from build123d import *

# Parameters (mm, degrees)
BASE_FLANGE1_DEPTH                 = 85.725
SKETCH2_R                          = 6.5532
SKETCH2_R_2                        = 3.3147
SKETCH2_R_3                        = 2.667
SKETCH2_R_4                        = 1.8669
FCE_1_INDICATOR_HOLES_DEPTH        = 2.54
SKETCH3_R                          = 2.1082
FCE_2_BRACKET_MOUNTING_HOLES_DEPTH = 2.54
CHAMFER1_SIZE                      = 1.27
SKETCH8_R                          = 2.1082
FCE_3_BOARD_MOUNTING_HOLES_DEPTH   = 2.54
FILLET1_R                          = 3.175


# Sheet-metal steps are written as plain solids
with BuildPart() as part:
    # Sketch1 → Base-Flange1 (new, symmetric)
    with BuildSketch(Plane(origin=(0, 0, 0), x_dir=(1, 0, 0), z_dir=(0, 1, 0))):
        with BuildLine():
            Line((-31.75, -101.6), (-3.302, -101.6))
            ThreePointArc((-3.302, -101.6), (-0.967133409, -100.632866591), (0, -98.298))
            Line((0, -98.298), (0, -3.302))
            ThreePointArc((0, -3.302), (-0.967133409, -0.967133409), (-3.302, 0))
            Line((-3.302, 0), (-53.975, 0))
            Line((-53.975, 0), (-53.975, -2.032))
            Line((-53.975, -2.032), (-3.302, -2.032))
            ThreePointArc((-3.302, -2.032), (-2.403974388, -2.403974388), (-2.032, -3.302))
            Line((-2.032, -3.302), (-2.032, -98.298))
            ThreePointArc((-2.032, -98.298), (-2.403974388, -99.196025612), (-3.302, -99.568))
            Line((-3.302, -99.568), (-31.75, -99.568))
            Line((-31.75, -99.568), (-31.75, -101.6))
        make_face()
    extrude(amount=BASE_FLANGE1_DEPTH, both=True)

    # Sketch2 → FCE-1 Indicator holes (cut)
    with BuildSketch(Plane(origin=(0, 0, 101.6), x_dir=(-1, 0, 0), z_dir=(0, 0, -1))):
        with Locations(Location((14.732, 63.5, 0), (0, 0, 180))):
            Circle(SKETCH2_R)
        with Locations(Location((14.732, 44.45, 0), (0, 0, 180))):
            Circle(SKETCH2_R)
        with Locations(Location((14.732, -12.7, 0), (0, 0, 180))):
            Circle(SKETCH2_R_2)
        with Locations(Location((18.034, -25.4, 0), (0, 0, 180))):
            Circle(SKETCH2_R_3)
        with Locations(Location((18.034, -38.1, 0), (0, 0, 180))):
            Circle(SKETCH2_R_3)
        with Locations(Location((18.034, -50.8, 0), (0, 0, 180))):
            Circle(SKETCH2_R_3)
        with Locations(Location((17.272, -63.5, 0), (0, 0, 180))):
            Circle(SKETCH2_R_4)
    extrude(amount=FCE_1_INDICATOR_HOLES_DEPTH, mode=Mode.SUBTRACT)

    # Sketch3 → FCE-2 Bracket Mounting Holes (cut)
    with BuildSketch(Plane.XY.offset(2.032)):
        with Locations((-44.45, 76.2)):
            Circle(SKETCH3_R)
        with Locations((-44.45, 0)):
            Circle(SKETCH3_R)
        with Locations((-44.45, -76.2)):
            Circle(SKETCH3_R)
    extrude(amount=-FCE_2_BRACKET_MOUNTING_HOLES_DEPTH, mode=Mode.SUBTRACT)

    # Chamfer1
    chamfer1_edges = [part.edges().sort_by_distance(p)[0] for p in [
        (-20.701, -25.4, 101.6),
        (-20.701, -38.1, 101.6),
        (-20.701, -50.8, 101.6),
    ]]
    chamfer(chamfer1_edges, length=CHAMFER1_SIZE)

    # Sketch8 → FCE-3 Board Mounting Holes (cut)
    with BuildSketch(Plane.ZY.offset(2.032)):
        with Locations((93.218, 76.2)):
            Circle(SKETCH8_R)
        with Locations((93.218, 0)):
            Circle(SKETCH8_R)
        with Locations((93.218, -76.2)):
            Circle(SKETCH8_R)
        with Locations((29.718, -76.2)):
            Circle(SKETCH8_R)
        with Locations((29.718, 0)):
            Circle(SKETCH8_R)
        with Locations((29.718, 76.2)):
            Circle(SKETCH8_R)
    extrude(amount=-FCE_3_BOARD_MOUNTING_HOLES_DEPTH, mode=Mode.SUBTRACT)

    # Fillet1
    fillet1_edges = [part.edges().sort_by_distance(p)[0] for p in [
        (-31.75, -85.725, 100.584),
        (-53.975, 85.725, 1.016),
        (-31.75, 85.725, 100.584),
        (-53.975, -85.725, 1.016),
    ]]
    fillet(fillet1_edges, radius=FILLET1_R)


solid = part.part
Can you work these out from the model? Positions are in its coordinate system, mm. A direction names the side the tool comes from. Coordinates: 2 decimals unless noted, no trailing zeros. Order: outer loops, then holes, each group sorted by start corner. A loop starts at its lowest first (then second) coordinate and runs counter-clockwise, first axis right, second up. Notation, with made-up numbers: M 18,-31.5 L 59,-31.5 A17 cw 59,-24.5 Z; hole C 73.25,23.25 d1. An arc over 180 degrees is marked long. Write item = value, one per line.
(1) Suppose I cut it at D-D on y = 44.45. Please give me the cut outline in (x, z) (3 decimals), plus the area to 3 significant figures.
Results are:
outline = M -53.975,0 L -3.302,0 A3.302 ccw 0,3.302 L 0,98.298 A3.302 ccw -3.302,101.6 L -8.179,101.6 L -8.179,99.568 L -3.302,99.568 A1.27 cw -2.032,98.298 L -2.032,3.302 A1.27 cw -3.302,2.032 L -53.975,2.032 Z; M -31.75,99.568 L -21.285,99.568 L -21.285,101.6 L -31.75,101.6 Z
area = 342 mm2
(2) For pin 1 Ø14 at (x, y) = (-14.5, -14) entering from -Z; pin 2 Ø3 at (x, y) = (-34, -65) entering from +Z; pin 3 Ø12 at (y, z) = (-39.5, 57.5) entering from -X; pin 4 Ø0.6 at (y, z) = (-22, 100.5) entering from -X, each with a flat end and sliding along its axis, tell me the tip position at first contact or that it passes through.
Results are:
pin_1 = 0
pin_2 = 2.03
pin_3 = -2.03
pin_4 = -31.75
(3) Suppose I cut it at A-A on y = 0. Please give me the cut outline in (x, z) (3 decimals).
Results are:
outline = M -53.975,0 L -46.558,0 L -46.558,2.032 L -53.975,2.032 Z; M -42.342,0 L -3.302,0 A3.302 ccw 0,3.302 L 0,27.61 L -2.032,27.61 L -2.032,3.302 A1.27 cw -3.302,2.032 L -42.342,2.032 Z; M -31.75,99.568 L -3.302,99.568 A1.27 cw -2.032,98.298 L -2.032,95.326 L 0,95.326 L 0,98.298 A3.302 ccw -3.302,101.6 L -31.75,101.6 Z; M -2.032,31.826 L 0,31.826 L 0,91.11 L -2.032,91.11 Z
(4) Suppose I cut it at C-C on x = -38.5. Please give me the cut outline in (y, z) (3 decimals), plus the area to 3 significant figures.
Results are:
outline = M -85.725,0 L 85.725,0 L 85.725,2.032 L -85.725,2.032 Z
area = 348 mm2
(5) If we mould it in two halves opening along X, with no side actions, what happens to faces 1 (the face through (-2.032, 1, 50)), 2 (the face through (-42.44, 0.63, 1.03)), 3 (the face through (-17, 1, 99.568))? For each: pulls with the +X half, pulls with the -X half, needs draft (parallel to the pull), parting line crosses it, or undercut.
Results are:
face_1 = pulls with the -X half
face_2 = undercut
face_3 = needs draft
(6) Suppose I cut it at B-B on y = -50.8. Please give me the cut outline in (x, z) (3 decimals).
Results are:
outline = M -53.975,0 L -3.302,0 A3.302 ccw 0,3.302 L 0,98.298 A3.302 ccw -3.302,101.6 L -14.097,101.6 L -15.367,100.33 L -15.367,99.568 L -3.302,99.568 A1.27 cw -2.032,98.298 L -2.032,3.302 A1.27 cw -3.302,2.032 L -53.975,2.032 Z; M -31.75,99.568 L -20.701,99.568 L -20.701,100.33 L -21.971,101.6 L -31.75,101.6 Z
(7) I need wall thicknesses on line 1 along Y through (x, z) = (-44.45, 0.85) (3 decimals); line 2 along Z through (x, y) = (-8, 6.5); line 3 along X through (y, z) = (50, 18). Which ranges of each line are inside material? Lowest first, please. Write a range as [from, to].
Results are:
line_1 = [-85.725, -78.308], [-74.092, -2.108], [2.108, 74.092], [78.308, 85.725]
line_2 = [0, 2.03], [99.57, 101.6]
line_3 = [-2.03, 0]
(8) For faces 4 (the face through (-1.03, 0.63, 31.73)), 5 (the face through (-30.795, -84.82, 100.598)), 6 (the face through (-16.803, -35.734, 99.954)), which set-ups out of +Z, -Z, +X, -X, +Y, -Y let a thin tool reach every point of the face, with its end or its side?
Results are:
face_4 = +X, -X
face_5 = +Z, -X, -Y
face_6 = +Z
